Could you check a few things on this drawing? It's one solid part, dimensions in mm from its lowest x, y, z. Give positions to 0.01 mm unless a question says otherwise; leave off trailing zeros. Loops run counter-clockwise (first coordinate to the right, second up) from the corner with the lowest first, then second, coordinate; pieces in that order, holes last.
1. I need wall thicknesses on line 1 along X through (y, z) = (1.7, 67.5); line 2 along X through (y, z) = (1.35, 95.25) (1 decimal). Which ranges of each line are inside material? Lowest first, please.
2. Imagine slicing it at C-C (z = 32). List the corners of the cut face in (x, y) for me (1 decimal).
3. Imagine slicing it at A-A (z = 6.35). List the corners of the cut face in (x, y) for me (1 decimal).
4. Imagine slicing it at B-B (x = 100.5). List the corners of the cut face in (y, z) for me (1 decimal).
5. Imagine slicing it at D-D (y = 2.15). Count the separate pieces of the cut face and the enclosed holes in it, plus the area to 3 significant figures.
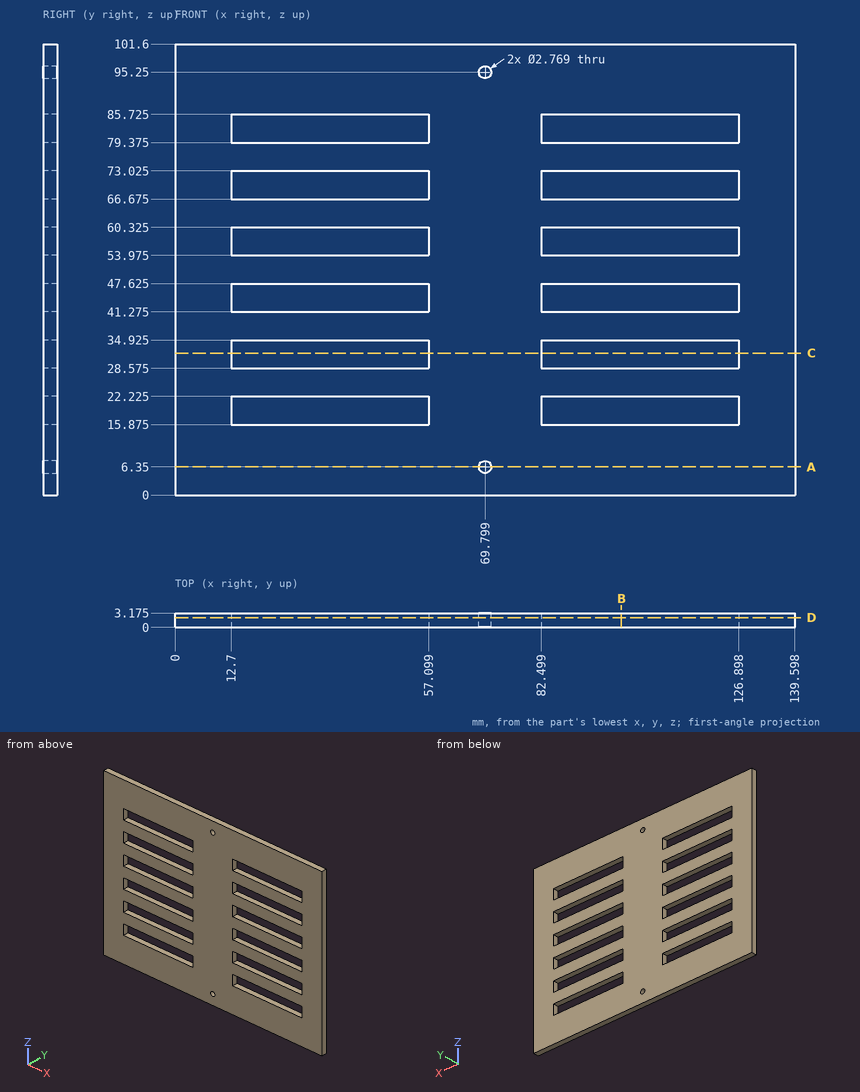
Derived:
1. line 1: x = 0 to 12.7, 57.1 to 82.5, 126.9 to 139.6
1. line 2: x = 0 to 68.4, 71.2 to 139.6
2. outline: (0, 0) - (12.7, 0) - (12.7, 3.2) - (0, 3.2) - close; (57.1, 0) - (82.5, 0) - (82.5, 3.2) - (57.1, 3.2) - close; (126.9, 0) - (139.6, 0) - (139.6, 3.2) - (126.9, 3.2) - close
3. outline: (0, 0) - (68.4, 0) - (68.4, 3.2) - (0, 3.2) - close; (71.2, 0) - (139.6, 0) - (139.6, 3.2) - (71.2, 3.2) - close
4. outline: (0, 0) - (3.2, 0) - (3.2, 15.9) - (0, 15.9) - close; (0, 22.2) - (3.2, 22.2) - (3.2, 28.6) - (0, 28.6) - close; (0, 34.9) - (3.2, 34.9) - (3.2, 41.3) - (0, 41.3) - close; (0, 47.6) - (3.2, 47.6) - (3.2, 54) - (0, 54) - close; (0, 60.3) - (3.2, 60.3) - (3.2, 66.7) - (0, 66.7) - close; (0, 73) - (3.2, 73) - (3.2, 79.4) - (0, 79.4) - close; (0, 85.7) - (3.2, 85.7) - (3.2, 101.6) - (0, 101.6) - close
5. separate pieces: 1
5. enclosed holes: 14
5. area: 10,800 mm2
